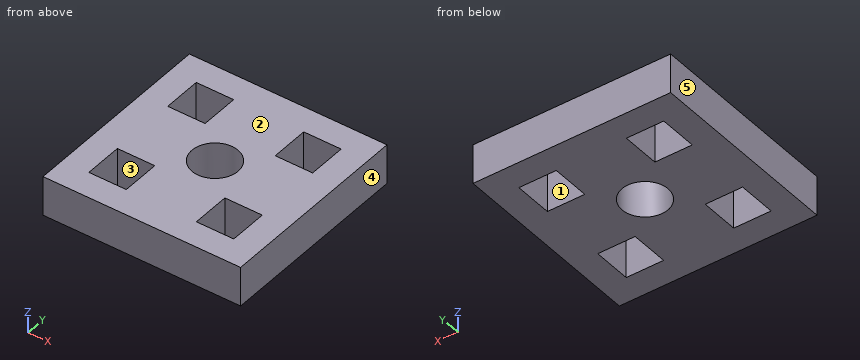
Autodesk Inventor part; units mm, degrees
ref_plane "YZ Plane" through (0, 0, 0) normal (1, 0, 0) x (0, 1, 0)
ref_plane "XZ Plane" through (0, 0, 0) normal (0, 1, 0) x (-1, 0, 0)
ref_plane "XY Plane" through (0, 0, 0) normal (0, 0, 1) x (1, 0, 0)
sketch "Sketch1" plane through (0, 0, 0) normal (0, 0, 1) x (1, 0, 0)
  line L0 (-7.5, -7.5) -> (7.5, -7.5)
  line L1 (7.5, -7.5) -> (7.5, 7.5)
  line L2 (7.5, 7.5) -> (-7.5, 7.5)
  line L3 (-7.5, 7.5) -> (-7.5, -7.5)
  line L4 (-7.5, -7.5) -> (7.5, 7.5) construction
  line L5 (7.5, -7.5) -> (-7.5, 7.5) construction
  line L6 (-5.5, 2.58) -> (-2.66, 2.58)
  line L7 (-2.66, 2.58) -> (-2.66, 5.5)
  line L8 (-2.66, 5.5) -> (-5.5, 5.5)
  line L9 (-5.5, 5.5) -> (-5.5, 2.58)
  line L10 (0, 0) -> (0, 4.08) construction
  line L11 (0, 0) -> (5.4269, 0) construction
  line L12 (2.66, 2.58) -> (2.66, 5.5)
  line L13 (2.66, 5.5) -> (5.5, 5.5)
  line L14 (5.5, 5.5) -> (5.5, 2.58)
  line L15 (5.5, 2.58) -> (2.66, 2.58)
  line L16 (2.66, -2.58) -> (2.66, -5.5)
  line L17 (5.5, -2.58) -> (2.66, -2.58)
  line L18 (5.5, -5.5) -> (5.5, -2.58)
  line L19 (2.66, -5.5) -> (5.5, -5.5)
  line L20 (-5.5, -2.58) -> (-2.66, -2.58)
  line L21 (-2.66, -5.5) -> (-5.5, -5.5)
  line L22 (-5.5, -5.5) -> (-5.5, -2.58)
  line L23 (-2.66, -2.58) -> (-2.66, -5.5)
  circle A0 centre (0, 0) radius 1.75
  dimension "d2" = 15
  dimension "d4" = 2.84
  dimension "d5" = 2.92
  dimension "d6" = 2
  dimension "d7" = 2
  dimension "d8" = 3.5
extrude "Extrusion1" add sketch "Sketch1" along normal blind 3
equation "\"d6\" = d7"
equation "\"d8\" = stickL"
equation "\"thick\" = 0.5"
equation "\"lrlr\" = 19"
equation "\"lrmid\" = 19.9"
equation "\"lrdepth\" = 3.3"
equation "\"mlr\" = 16.6"
equation "\"mmid\" = 24.7"
equation "\"mdepth\" = 4.5"
equation "\"lrltotal\" = 126.6"
equation "\"mltotal\" = 126.6"
equation "\"lrbetween\" = 52.1"
equation "\"mbetween\" = 49.5"
equation "\"toler\" = 1"
equation "\"tight\" = 0.08"
equation "\"stuckw\" = 6"
equation "\"sidewallL\" = 132.6"
equation "\"heaterH\" = 117.3"
equation "\"stickL\" = 3.5"
equation "\"wireH\" = 25"
properties part number "motor_top"
The listing builds one solid part. Answer for the finished solid, in the listing's coordinates (mm). Face numbers are marked on the shaded views. A direction names the side the tool comes from. Coordinates: 2 decimals unless noted, no trailing zeros. Loops run counter-clockwise (first coordinate to the right, second up) from the corner with the lowest first, then second, coordinate; pieces in that order, holes last. Notation, with made-up numbers: (53.25, 65.5) -> (112.25, 65.5) arc R10 ccw to (112.25, 77.5) -> close; hole circle Ø3 at (30, 22.25). An arc over 180 degrees is marked (long way). Use one line per item in the form item = value. Start each with the question number.
Item 1: A tool of negligible diameter and unlimited length cuts with its end or side. For the marked faces 1 and 2, from which of +Z, -Z, +X, -X, +Y, -Y can it reach the whole face along a straight path? Write none if from no direction.
Item 2: The part is cut by section C-C on z = 1.45. Determine the outline of the cut face in (x, y).
Item 3: The part is cut by section B-B on x = -4.75. Determine the outline of the cut face in (y, z).
Item 4: The mould has two halves that part along X. Classify the marked faces 3, 4 and 5: released by +X, released by -X, zero draft, split by the parting line, or undercut.
Item 5: The part is cut by section A-A on y = 3.25. Determine the outline of the cut face in (x, z).
Item 6: The part is cut by section D-D on y = 0. Determine the outline of the cut face in (x, z).
Item 7: Consider L1, parallel to X at y = -3.75, z = 1.25; L2, parallel to Y at x = 3.5, z = 0.3; L3, parallel to Y at x = 0, z = 1.1. Determine where each line is inside the solid, lowest interval first. Write a range as [from, to].
Answer key:
q1.face_1 = +Z, -Z
q1.face_2 = +Z, +X, -X, +Y, -Y
q2.outline = (-7.5, -7.5) -> (7.5, -7.5) -> (7.5, 7.5) -> (-7.5, 7.5) -> close; hole (-5.5, -5.5) -> (-2.66, -5.5) -> (-2.66, -2.58) -> (-5.5, -2.58) -> close; hole (-5.5, 2.58) -> (-2.66, 2.58) -> (-2.66, 5.5) -> (-5.5, 5.5) -> close; hole circle Ø3.5 at (0, 0); hole (2.66, -5.5) -> (5.5, -5.5) -> (5.5, -2.58) -> (2.66, -2.58) -> close; hole (2.66, 2.58) -> (5.5, 2.58) -> (5.5, 5.5) -> (2.66, 5.5) -> close
q3.outline = (-7.5, 0) -> (-5.5, 0) -> (-5.5, 3) -> (-7.5, 3) -> close; (-2.58, 0) -> (2.58, 0) -> (2.58, 3) -> (-2.58, 3) -> close; (5.5, 0) -> (7.5, 0) -> (7.5, 3) -> (5.5, 3) -> close
q4.face_3 = undercut
q4.face_4 = released by +X
q4.face_5 = released by -X
q5.outline = (-7.5, 0) -> (-5.5, 0) -> (-5.5, 3) -> (-7.5, 3) -> close; (-2.66, 0) -> (2.66, 0) -> (2.66, 3) -> (-2.66, 3) -> close; (5.5, 0) -> (7.5, 0) -> (7.5, 3) -> (5.5, 3) -> close
q6.outline = (-7.5, 0) -> (-1.75, 0) -> (-1.75, 3) -> (-7.5, 3) -> close; (1.75, 0) -> (7.5, 0) -> (7.5, 3) -> (1.75, 3) -> close
q7.L1 = [-7.5, -5.5], [-2.66, 2.66], [5.5, 7.5]
q7.L2 = [-7.5, -5.5], [-2.58, 2.58], [5.5, 7.5]
q7.L3 = [-7.5, -1.75], [1.75, 7.5]
